from build123d import *

# Parameters (mm, degrees)
SKETCH1_W           = 38.1
SKETCH1_H           = 12.7
BOSS_EXTRUDE1_DEPTH = 615.95
SKETCH2_R           = 14.3002
CUT_EXTRUDE1_DEPTH  = 762
SKETCH3_W           = 38.1
SKETCH3_H           = 12.7
BOSS_EXTRUDE2_DEPTH = 38.1
SKETCH4_R           = 14.3002
CUT_EXTRUDE2_DEPTH  = 101.6


with BuildPart() as part:
    # Sketch1 → Boss-Extrude1 (new body)
    with BuildSketch(Plane.XY):
        with Locations((19.05, 6.35)):
            Rectangle(SKETCH1_W, SKETCH1_H)
    extrude(amount=BOSS_EXTRUDE1_DEPTH)

    # Sketch2 → Cut-Extrude1 (cut)
    with BuildSketch(Plane(origin=(0, 12.7, 0), x_dir=(1, 0, 0), z_dir=(0, 1, 0))):
        with Locations((19.05, -588.9498)):
            Circle(SKETCH2_R)
        with Locations((19.05, -27.0002)):
            Circle(SKETCH2_R)
    extrude(amount=-CUT_EXTRUDE1_DEPTH, mode=Mode.SUBTRACT)

    # Sketch3 → Boss-Extrude2 (add)
    with BuildSketch(Plane(origin=(0, 0, 0), x_dir=(-1, 0, 0), z_dir=(0, 0, -1))):
        with Locations((-19.05, 6.35)):
            Rectangle(SKETCH3_W, SKETCH3_H)
    extrude(amount=BOSS_EXTRUDE2_DEPTH)

    # Sketch4 → Cut-Extrude2 (cut)
    with BuildSketch(Plane(origin=(0, 12.7, 0), x_dir=(1, 0, 0), z_dir=(0, 1, 0))):
        with Locations((19.05, 19.0373)):
            Circle(SKETCH4_R)
    extrude(amount=-CUT_EXTRUDE2_DEPTH, mode=Mode.SUBTRACT)


solid = part.part
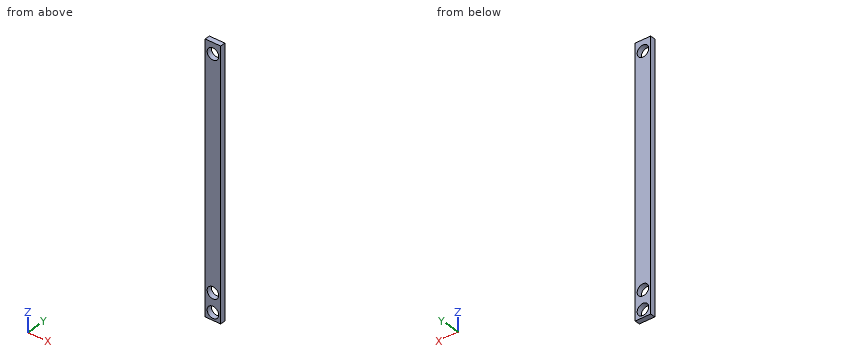
Work out the finished part from the listing and answer in its coordinate system (mm). Round coordinates to 2 decimals unless told otherwise and drop trailing zeros. Loops run counter-clockwise (first coordinate to the right, second up) from the corner with the lowest first, then second, coordinate; pieces in that order, holes last. Notation, with made-up numbers: M 36,-6 L 48,-6 A17 cw 48,2 Z; hole C 49,44 d8. An arc over 180 degrees is marked long. One line per question, with ' | ' between items. Start each with the question number.
(1) Find the intervals of material crossed by line 1 (Z direction, x = 19.05, y = 9.5); line 2 (Z direction, x = 18, y = 5.25), in increasing order.
(2) A cutting plane is placed at A-A on x = 19.05. Write down the section's boundary in (y, z).
(3) A flat-ended cylindrical pin translates along its axis: pin 1 Ø17 at (x, z) = (19.05, 588.95) entering from -Y. Find the tip coordinate at first contact, or state that the pin passes through.
(4) A cutting plane is placed at B-B on y = 5.25. Write down the section's boundary in (x, z), plus the area to 3 significant figures.
Geometry check:
1) line 1: z = -38.1 to -33.34, -4.74 to 12.7, 41.3 to 574.65, 603.25 to 615.95 | line 2: z = -38.1 to -33.3, -4.78 to 12.74, 41.26 to 574.69, 603.21 to 615.95
2) outline: M 0,-38.1 L 12.7,-38.1 L 12.7,-33.34 L 0,-33.34 Z; M 0,-4.74 L 12.7,-4.74 L 12.7,12.7 L 0,12.7 Z; M 0,41.3 L 12.7,41.3 L 12.7,574.65 L 0,574.65 Z; M 0,603.25 L 12.7,603.25 L 12.7,615.95 L 0,615.95 Z
3) pin 1: passes through
4) outline: M 0,-38.1 L 38.1,-38.1 L 38.1,615.95 L 0,615.95 Z; hole C 19.05,-19.04 d28.6; hole C 19.05,27 d28.6; hole C 19.05,588.95 d28.6 | area: 23,000 mm²
